Check sheet for the drawn part. Datum: minimum x, y, z corner. Units: mm. Round coordinates to 2 decimals unless told otherwise and drop trailing zeros. Write each loop counter-clockwise with the first axis right and the second up, starting at its lowest first coordinate (ties: lowest second). Pieces come first, ordered by that corner, then holes. Notation, with made-up numbers: (12, 37) -> (30, 37) arc R8 ccw to (30, 44) -> close; hole circle Ø1 at (82.5, 17). An arc over 180 degrees is marked (long way). One line per item, written item: value.
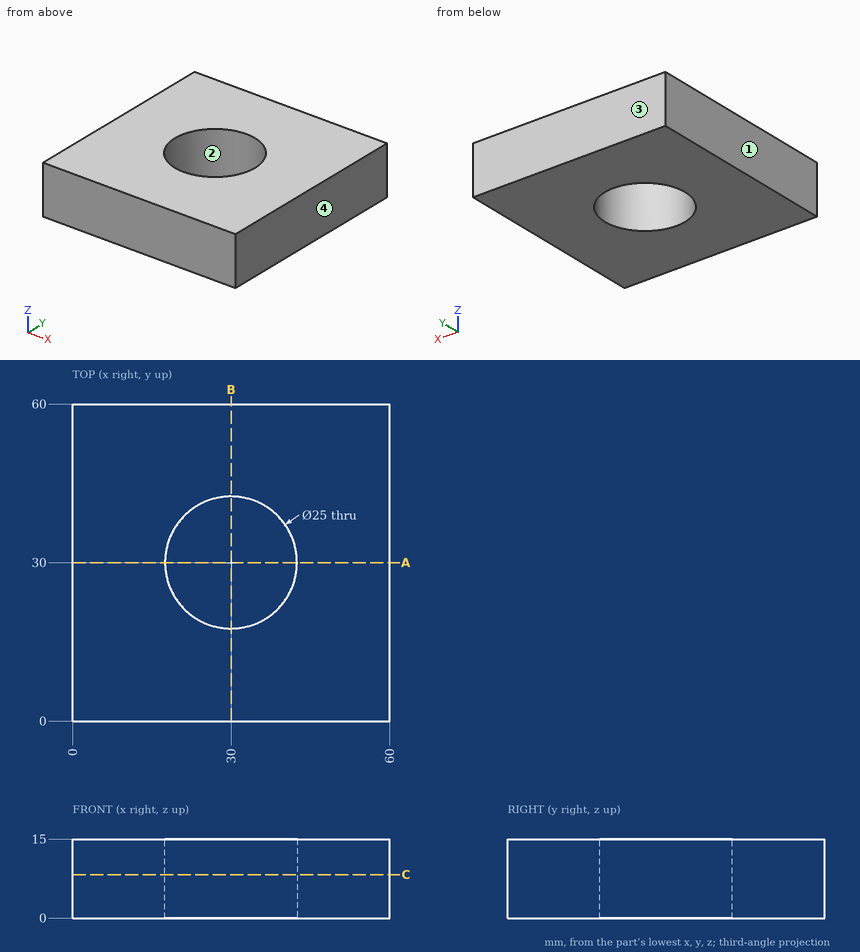
Item 1: Thickness scan on line 1 (Y direction, x = 30, z = 7.5); line 2 (Y direction, x = 24.5, z = 2.25); line 3 (X direction, y = 41, z = 13.75). Record the ranges inside material, lowest first.
Answer:
line 1: y = 0 to 17.5, 42.5 to 60
line 2: y = 0 to 18.78, 41.22 to 60
line 3: x = 0 to 24.06, 35.94 to 60
Item 2: Sectioned sample at C-C on z = 8.25. Enter the section's corners in (x, y).
Answer:
outline: (0, 0) -> (60, 0) -> (60, 60) -> (0, 60) -> close; hole circle Ø25 at (30, 30)
Item 3: Mould release check, pull along X, two halves, no side actions. Record for the marked faces 1, 2, 3 and 4: pulls with the +X half, pulls with the -X half, needs draft (parallel to the pull), parting line crosses it, or undercut.
Answer:
face 1: pulls with the -X half
face 2: undercut
face 3: needs draft
face 4: pulls with the +X half
Item 4: Depth check by flat-ended pin: P1, Ø8, axis at x = 12.5, z = 7.5, coming from the -Y side. Enter the tip coordinate at first touch or a pass-through.
Answer:
P1: stops at y = 0
Item 5: Sectioned sample at A-A on y = 30. Enter the section's corners in (x, z).
Answer:
outline: (0, 0) -> (17.5, 0) -> (17.5, 15) -> (0, 15) -> close; (42.5, 0) -> (60, 0) -> (60, 15) -> (42.5, 15) -> close
